from build123d import *

# Parameters (mm, degrees)
BOSS_EXTRUDE1_DEPTH = 10
SKETCH2_R           = 11
CUT_EXTRUDE1_DEPTH  = 10


with BuildPart() as part:
    # Sketch1 → Boss-Extrude1 (new body)
    with BuildSketch(Plane.XY):
        Polygon((50, 20), (50, 100), (10, 100), (10, 20), (0, 20), (0, 0), (60, 0), (60, 20), align=None)
        with BuildLine():
            Line((50, 100), (10, 100))
            ThreePointArc((10, 100), (30, 120), (50, 100))
        make_face()
    extrude(amount=BOSS_EXTRUDE1_DEPTH)

    # Sketch2 → Cut-Extrude1 (cut)
    with BuildSketch(Plane.XY.offset(10)):
        with Locations((30, 100)):
            Circle(SKETCH2_R)
    extrude(amount=-CUT_EXTRUDE1_DEPTH, mode=Mode.SUBTRACT)


solid = part.part
Model file for the job. Use its own axes, mm. A direction names the side the tool comes from. Give positions to 0.01 mm unless a question says otherwise; leave off trailing zeros. Write each loop counter-clockwise with the first axis right and the second up, starting at its lowest first coordinate (ties: lowest second). Pieces come first, ordered by that corner, then holes. Notation, with made-up numbers: M -17,38.5 L 30,38.5 A19 ccw 30,44.5 Z; hole C 57.5,45.5 d11. An arc over 180 degrees is marked long. One line per item, written item: value. Start each with the question number.
Q1. Saw through at B-B, the plane x = 30. Write the cut outline in (y, z), plus the area to 3 significant figures.
Q2. Drop flat-ended pins along their axis: pin 1 Ø5 at (y, z) = (60, 3) entering from +X; pin 2 Ø3 at (x, z) = (49.5, 3) entering from +Y; pin 3 Ø20 at (x, y) = (30, 100) entering from +Z; pin 4 Ø3 at (x, z) = (55, 4) entering from +Y. Give the stop position or say it passes through.
Q3. Saw through at D-D, the plane y = 72. Write the cut outline in (x, z), plus the area to 3 significant figures.
Q4. Two-plate mould, pull along X, no slides. Class faces 4 (the cylindrical face through (28.568, 110.906, 5.07)), 5 (the flat face through (50, 59, 5)), 6 (the flat face through (30, 0, 5)), 7 (the flat face through (0, 10, 5)): +X half, -X half, draft (parallel to the pull), parting line (faces both ways), or undercut.
Q5. Saw through at A-A, the plane z = 7.25. Write the cut outline in (x, y), plus the area to 3 significant figures.
Q6. Saw through at C-C, the plane x = 21.5. Write the cut outline in (y, z).
Q7. 3-axis set-ups, long thin cutter, end or side, ignore diameter. For faces 1 (the cylindrical face through (30, 120, 5)), 2 (the flat face through (55, 20, 5)), 3 (the flat face through (10, 61, 5)): which of +Z, -Z, +X, -X, +Y, -Y reach the whole face in a straight line?
Q8. Probe probe 1 along Y at (x, z) = (30, 6); probe 2 along X at (y, z) = (39.5, 3); probe 3 along Y at (x, z) = (52, 3). List the from-to ranges inside material, lowest first. Write a range as [from, to].
Output values:
1. outline: M 0,0 L 89,0 L 89,10 L 0,10 Z; M 111,0 L 120,0 L 120,10 L 111,10 Z
1. area: 980 mm²
2. pin 1: stops at x = 50
2. pin 2: stops at y = 108.72
2. pin 3: passes through
2. pin 4: stops at y = 20
3. outline: M 10,0 L 50,0 L 50,10 L 10,10 Z
3. area: 400 mm²
4. face 4: undercut
4. face 5: +X half
4. face 6: draft
4. face 7: -X half
5. outline: M 0,0 L 60,0 L 60,20 L 50,20 L 50,100 A20 ccw 10,100 L 10,20 L 0,20 Z; hole C 30,100 d22
5. area: 4,650 mm²
6. outline: M 0,0 L 93.02,0 L 93.02,10 L 0,10 Z; M 106.98,0 L 118.1,0 L 118.1,10 L 106.98,10 Z
7. face 1: +Z, -Z, +Y
7. face 2: +Z, -Z, +X, +Y
7. face 3: +Z, -Z, -X, +Y
8. probe 1: y = [0, 89], [111, 120]
8. probe 2: x = [10, 50]
8. probe 3: y = [0, 20]
